Design review of the part built by this model. Coordinates are the model's own, in mm. A direction names the side the tool comes from. Coordinates: 2 decimals unless noted, no trailing zeros. Loops run counter-clockwise (first coordinate to the right, second up) from the corner with the lowest first, then second, coordinate; pieces in that order, holes last. Notation, with made-up numbers: (-31, -20.75) -> (14, -20.75) arc R19 cw to (14, 11.25) -> close; hole circle Ø2 at (-5.5, -36.5). An arc over 180 degrees is marked (long way). Answer in a Markdown table with one row per item.
```python
from build123d import *

# Parameters (mm, degrees)
F1_R          = 1.25
F2_DEPTH      = 12.0689655172
F3_W          = 13.7931034483
F3_H          = 9.1954022989
F4_DEPTH      = 8.0469770115
F5_W          = 4
F5_H          = 5.0459770115
F5_R          = 1
F6_DEPTH      = 8.0459770115
F6_DEPTH_BACK = 1.4942528736
F7_W          = 4
F7_H          = 5.0459770115
F7_R          = 1
F8_DEPTH      = 12.9885057471
F8_DEPTH_BACK = 8.0459770115


with BuildPart() as f2:
    # F1 (on Front) → F2 (new body)
    with BuildSketch(Plane.XZ):
        Polygon((-17.2413793103, 0), (0, 0), (17.2413793103, 0), (17.2413793103, 1.724137931), (17.2413793103, 8.0459770115), (0, 8.0459770115), (-17.2413793103, 8.0459770115), (-17.2413793103, 1.724137931), align=None)
        with Locations((-8.6206896552, 4.2873563218)):
            Circle(F1_R, mode=Mode.SUBTRACT)
        with Locations((8.6206896552, 4.2873563218)):
            Circle(F1_R, mode=Mode.SUBTRACT)
    extrude(amount=F2_DEPTH)

    # F3 (on face) → F4 (cut, through all)
    with BuildSketch(Plane.XY.offset(8.0459770115)):
        with Locations((-8.0459770115, -6.0344827586)):
            Rectangle(F3_W, F3_H)
        with Locations((8.0459770115, -6.0344827586)):
            Rectangle(F3_W, F3_H)
    extrude(amount=-F4_DEPTH, mode=Mode.SUBTRACT)

    # F5 (on face) → F6 (join, two sides)
    with BuildSketch(Plane(origin=(0, 0, 0), x_dir=(1, 0, 0), z_dir=(0, 0, -1))) as f6_sk:
        with Locations((-14.367816092, 14.591954023)):
            Rectangle(F5_W, F5_H)
        with Locations((-14.367816092, 15.1149425287)):
            Circle(F5_R, mode=Mode.SUBTRACT)
        with Locations((14.367816092, 14.591954023)):
            Rectangle(F5_W, F5_H)
        with Locations((14.367816092, 15.1149425287)):
            Circle(F5_R, mode=Mode.SUBTRACT)
        with Locations((-14.367816092, -2.5229885057)):
            Rectangle(F5_W, F5_H)
        with Locations((-14.367816092, -3.0459770115)):
            Circle(F5_R, mode=Mode.SUBTRACT)
        with Locations((14.367816092, -2.5229885057)):
            Rectangle(F5_W, F5_H)
        with Locations((14.367816092, -3.0459770115)):
            Circle(F5_R, mode=Mode.SUBTRACT)
    extrude(amount=-F6_DEPTH)
    extrude(f6_sk.sketch, amount=F6_DEPTH_BACK)

    # F7 (on face) → F8 (join, two sides)
    with BuildSketch(Plane(origin=(0, 0, 0), x_dir=(1, 0, 0), z_dir=(0, 0, -1))) as f8_sk:
        with Locations((0, 14.591954023)):
            Rectangle(F7_W, F7_H)
        with Locations((0, 15.1149425287)):
            Circle(F7_R, mode=Mode.SUBTRACT)
        with Locations((0, -2.5229885057)):
            Rectangle(F7_W, F7_H)
        with Locations((0, -3.0459770115)):
            Circle(F7_R, mode=Mode.SUBTRACT)
    extrude(amount=F8_DEPTH)
    extrude(f8_sk.sketch, amount=-F8_DEPTH_BACK)


solid = f2.part
```
(1) Take a section at C-C on z = -10. Give the boundary of the cut face in (x, y).
Evaluation:
| item | result |
|---|---|
| outline | (-2, -17.11) -> (2, -17.11) -> (2, -12.07) -> (-2, -12.07) -> close; (-2, 0) -> (2, 0) -> (2, 5.05) -> (-2, 5.05) -> close; hole circle Ø2 at (0, -15.11); hole circle Ø2 at (0, 3.05) |
(2) To check wall thickness, follow probe 1 along Y at (x, z) = (0, -5); probe 2 along X at (y, z) = (-2, 1); probe 3 along X at (y, z) = (-15, -5.5). State the ranges of each line that lie inside material, in increasing order.
Evaluation:
| item | result |
|---|---|
| probe 1 | y = -17.11 to -16.11, -14.11 to -12.07, 0 to 2.05, 4.05 to 5.05 |
| probe 2 | x = -17.24 to -14.94, -1.15 to 1.15, 14.94 to 17.24 |
| probe 3 | x = -2 to -0.99, 0.99 to 2 |
(3) Tool access review of faces 4 (the flat face through (-12.368, 3, 3)), 5 (the flat face through (0, 0, -6)), 6 (the flat face through (12.368, -15, 3)): name each direction out of +Z, -Z, +X, -X, +Y, -Y from which nothing blocks a thin tool from reaching the whole face with its end or side.
Evaluation:
| item | result |
|---|---|
| face 4 | +Z, -Z, +Y |
| face 5 | -Z, +X, -X |
| face 6 | +Z, -Z, -Y |
(4) Draft analysis for pull direction Z (two halves, no side actions). For faces 1 (the cylindrical face through (7.629, -11.341, 3.527)), 2 (the flat face through (-7, -1.437, 4)), 3 (the flat face through (0, -6, 8.046)), state which applies: pulls with the +Z half, pulls with the -Z half, needs draft (parallel to the pull), parting line crosses it, or undercut.
Evaluation:
| item | result |
|---|---|
| face 1 | undercut |
| face 2 | needs draft |
| face 3 | pulls with the +Z half |
(5) Take a section at B-B on x = -11. Give the boundary of the cut face in (y, z).
Evaluation:
| item | result |
|---|---|
| outline | (-12.07, 0) -> (-10.63, 0) -> (-10.63, 8.05) -> (-12.07, 8.05) -> close; (-1.44, 0) -> (0, 0) -> (0, 8.05) -> (-1.44, 8.05) -> close |
(6) Take a section at A-A on x = 0. Give the boundary of the cut face in (y, z).
Evaluation:
| item | result |
|---|---|
| outline | (-17.11, -12.99) -> (-16.11, -12.99) -> (-16.11, 8.05) -> (-17.11, 8.05) -> close; (-14.11, -12.99) -> (-12.07, -12.99) -> (-12.07, 0) -> (0, 0) -> (0, -12.99) -> (2.05, -12.99) -> (2.05, 8.05) -> (-14.11, 8.05) -> close; (4.05, -12.99) -> (5.05, -12.99) -> (5.05, 8.05) -> (4.05, 8.05) -> close |
(7) For pin 1 (1.5 mm diameter, centred on x = 7.5, y = -9, fed in from -Z); pin 2 (2.5 mm diameter, centred on x = -9, z = 3.5, fed in from +Y); pin 3 (6.5 mm diameter, centred on x = 7.5, z = 6, fed in from -Y); pin 4 (1.5 mm diameter, centred on x = -12, y = 0.5, fed in from -Z), all flat-tipped, find the tip position at first contact; note any pin that passes through.
Evaluation:
| item | result |
|---|---|
| pin 1 | passes through |
| pin 2 | stops at y = 0 |
| pin 3 | stops at y = -12.07 |
| pin 4 | stops at z = -1.49 |
(8) Take a section at D-D on y = -13.5. Give the boundary of the cut face in (x, z).
Evaluation:
| item | result |
|---|---|
| outline | (-16.37, -1.49) -> (-12.37, -1.49) -> (-12.37, 8.05) -> (-16.37, 8.05) -> close; (-2, -12.99) -> (2, -12.99) -> (2, 8.05) -> (-2, 8.05) -> close; (12.37, -1.49) -> (16.37, -1.49) -> (16.37, 8.05) -> (12.37, 8.05) -> close |
